Could you check a few things on this model? Use its own coordinates, in mm. A direction names the side the tool comes from. Give positions to 0.01 mm unless a question says otherwise; leave off trailing zeros. Write each loop counter-clockwise with the first axis right and the second up, starting at its lowest first coordinate (ties: lowest second). Pieces come first, ordered by that corner, then holes. Notation, with made-up numbers: (16.25, 8) - (34.25, 8) arc R23 ccw to (34.25, 27) - close; hole circle Ø2 at (42, 50.5). An arc over 180 degrees is marked (long way). Answer in a Markdown table with one row per item.
from build123d import *

# Parameters (mm, degrees)
BOSS_EXTRUDE1_DEPTH          = 6
CHAMFER1_SIZE                = 5
BOSS_EXTRUDE2_DEPTH          = 3
CHAMFER2_SIZE                = 3
SKETCH3_R                    = 2.55
CUT_EXTRUDE1_DEPTH           = 72.316197319
BOSS_EXTRUDE3_START          = 6
SKETCH4_R                    = 5
SKETCH4_R_2                  = 2.55
BOSS_EXTRUDE3_DEPTH          = 6
CHAMFER3_SIZE                = 1
CHAMFER4_SIZE                = 0.5
SKETCH5_R                    = 4.1
CUT_EXTRUDE2_DEPTH           = 5
SKETCH6_R                    = 2.6
CUT_EXTRUDE3_DEPTH           = 10
SKETCH7_R                    = 5
CUT_EXTRUDE4_DEPTH           = 2.8
CUT_EXTRUDE4_DRAFT           = -45
CUT_EXTRUDE4_PROFILE_2_DEPTH = 2.8
CUT_EXTRUDE4_PROFILE_2_DRAFT = -45
CUT_EXTRUDE4_PROFILE_3_DEPTH = 2.8
CUT_EXTRUDE4_PROFILE_3_DRAFT = -45
CUT_EXTRUDE4_PROFILE_4_DEPTH = 2.8
CUT_EXTRUDE4_PROFILE_4_DRAFT = -45
FILLET1_R                    = 2
CUT_EXTRUDE5_START           = -3
SKETCH8_W                    = 20
SKETCH8_H                    = 10
CUT_EXTRUDE5_DEPTH           = 10
CHAMFER5_SIZE                = 2
SKETCH9_R                    = 1.55
SKETCH9_W                    = 3
SKETCH9_H                    = 10
CUT_EXTRUDE6_DEPTH           = 10


with BuildPart() as part:
    # Sketch1 → Boss-Extrude1 (new body)
    with BuildSketch(Plane(origin=(0, 0, 0), x_dir=(1, 0, 0), z_dir=(0, 1, 0))):
        with BuildLine():
            Line((-32, -55), (32, -55))
            ThreePointArc((32, -55), (41.192388155, -51.192388155), (45, -42))
            Line((45, -42), (45, 42))
            ThreePointArc((45, 42), (41.192388155, 51.192388155), (32, 55))
            Line((32, 55), (-32, 55))
            ThreePointArc((-32, 55), (-41.192388155, 51.192388155), (-45, 42))
            Line((-45, 42), (-45, -42))
            ThreePointArc((-45, -42), (-41.192388155, -51.192388155), (-32, -55))
        make_face()
    extrude(amount=BOSS_EXTRUDE1_DEPTH)

    # Chamfer1
    chamfer1_edges = [part.edges().sort_by_distance(p)[0] for p in [
        (45, 0, 0),
        (41.192388155, 0, 51.192388155),
        (0, 0, 55),
        (-41.192388155, 0, 51.192388155),
        (-45, 0, 0),
        (-41.192388155, 0, -51.192388155),
        (0, 0, -55),
        (41.192388155, 0, -51.192388155),
    ]]
    chamfer(chamfer1_edges, length=CHAMFER1_SIZE)

    # Sketch2 → Boss-Extrude2 (add)
    with BuildSketch(Plane(origin=(0, 6, 0), x_dir=(1, 0, 0), z_dir=(0, 1, 0))):
        with BuildLine():
            ThreePointArc((-37.9, -42), (-36.171930009, -46.171930009), (-32, -47.9))
            Line((-32, -47.9), (32, -47.9))
            ThreePointArc((32, -47.9), (36.171930009, -46.171930009), (37.9, -42))
            Line((37.9, -42), (37.9, -21))
            Line((37.9, -21), (41.9, -21))
            Line((41.9, -21), (41.9, -42))
            ThreePointArc((41.9, -42), (39.000357134, -49.000357134), (32, -51.9))
            Line((32, -51.9), (-32, -51.9))
            ThreePointArc((-32, -51.9), (-39.000357134, -49.000357134), (-41.9, -42))
            Line((-41.9, -42), (-41.9, -21))
            Line((-41.9, -21), (-37.9, -21))
            Line((-37.9, -21), (-37.9, -42))
        make_face()
        with BuildLine():
            ThreePointArc((-41.9, 42), (-39.000357134, 49.000357134), (-32, 51.9))
            Line((-32, 51.9), (32, 51.9))
            ThreePointArc((32, 51.9), (39.000357134, 49.000357134), (41.9, 42))
            Line((41.9, 42), (41.9, 21))
            Line((41.9, 21), (37.9, 21))
            Line((37.9, 21), (37.9, 42))
            ThreePointArc((37.9, 42), (36.171930009, 46.171930009), (32, 47.9))
            Line((32, 47.9), (-32, 47.9))
            ThreePointArc((-32, 47.9), (-36.171930009, 46.171930009), (-37.9, 42))
            Line((-37.9, 42), (-37.9, 21))
            Line((-37.9, 21), (-41.9, 21))
            Line((-41.9, 21), (-41.9, 42))
        make_face()
    extrude(amount=BOSS_EXTRUDE2_DEPTH)

    # Chamfer2
    chamfer2_edges = [part.edges().sort_by_distance(p)[0] for p in [
        (37.9, 9, 31.5),
        (36.171930009, 9, 46.171930009),
        (0, 9, 47.9),
        (-36.171930009, 9, 46.171930009),
        (-37.9, 9, 31.5),
        (-37.9, 9, -31.5),
        (-36.171930009, 9, -46.171930009),
        (0, 9, -47.9),
        (36.171930009, 9, -46.171930009),
        (37.9, 9, -31.5),
    ]]
    chamfer(chamfer2_edges, length=CHAMFER2_SIZE - 0.0001)  # a hair under: the kernel refuses the full size

    # Sketch3 → Cut-Extrude1 (cut, through all)
    with BuildSketch(Plane(origin=(0, 6, 0), x_dir=(1, 0, 0), z_dir=(0, 1, 0))):
        with Locations(Location((-25, 30.5, 0), (0, 0, 270))):
            Circle(SKETCH3_R)
        with Locations(Location((25, 30.5, 0), (0, 0, 90))):
            Circle(SKETCH3_R)
        with Locations(Location((25, -30.5, 0), (0, 0, 270))):
            Circle(SKETCH3_R)
        with Locations(Location((-25, -30.5, 0), (0, 0, 90))):
            Circle(SKETCH3_R)
    extrude(amount=-CUT_EXTRUDE1_DEPTH, mode=Mode.SUBTRACT)

    # Sketch4 → Boss-Extrude3 (add)
    # profile 1 of 4: a face of its own
    with BuildSketch(Plane(origin=(0, 6, 0), x_dir=(1, 0, 0), z_dir=(0, 1, 0)).offset(BOSS_EXTRUDE3_START)):
        with Locations(Location((-25, -30.5, 0), (0, 0, 90))):
            Circle(SKETCH4_R)
        with Locations(Location((-25, -30.5, 0), (0, 0, 270))):
            Circle(SKETCH4_R_2, mode=Mode.SUBTRACT)
    # profile 2 of 4: a face of its own
    with BuildSketch(Plane(origin=(0, 6, 0), x_dir=(1, 0, 0), z_dir=(0, 1, 0)).offset(BOSS_EXTRUDE3_START)):
        with Locations(Location((25, -30.5, 0), (0, 0, 90))):
            Circle(SKETCH4_R)
        with Locations(Location((25, -30.5, 0), (0, 0, 270))):
            Circle(SKETCH4_R_2, mode=Mode.SUBTRACT)
    # profile 3 of 4: a face of its own
    with BuildSketch(Plane(origin=(0, 6, 0), x_dir=(1, 0, 0), z_dir=(0, 1, 0)).offset(BOSS_EXTRUDE3_START)):
        with Locations(Location((-25, 30.5, 0), (0, 0, 90))):
            Circle(SKETCH4_R)
        with Locations(Location((-25, 30.5, 0), (0, 0, 270))):
            Circle(SKETCH4_R_2, mode=Mode.SUBTRACT)
    # profile 4 of 4: a face of its own
    with BuildSketch(Plane(origin=(0, 6, 0), x_dir=(1, 0, 0), z_dir=(0, 1, 0)).offset(BOSS_EXTRUDE3_START)):
        with Locations(Location((25, 30.5, 0), (0, 0, 90))):
            Circle(SKETCH4_R)
        with Locations(Location((25, 30.5, 0), (0, 0, 270))):
            Circle(SKETCH4_R_2, mode=Mode.SUBTRACT)
    extrude(amount=-BOSS_EXTRUDE3_DEPTH)

    # Chamfer3
    chamfer3_edges = [part.edges().sort_by_distance(p)[0] for p in [
        (-25, 6, 35.5),
        (25, 6, 35.5),
        (-25, 6, -25.5),
        (25, 6, -25.5),
    ]]
    chamfer(chamfer3_edges, length=CHAMFER3_SIZE)

    # Chamfer4
    chamfer4_edges = [part.edges().sort_by_distance(p)[0] for p in [
        (-25, 12, 35.5),
        (25, 12, 35.5),
        (-25, 12, -25.5),
        (25, 12, -25.5),
    ]]
    chamfer(chamfer4_edges, length=CHAMFER4_SIZE)

    # Sketch5 → Cut-Extrude2 (cut)
    with BuildSketch(Plane.XZ):
        with Locations(Location((-25, 30.5, 0), (0, 0, 270))):
            Circle(SKETCH5_R)
        with Locations(Location((25, 30.5, 0), (0, 0, 270))):
            Circle(SKETCH5_R)
        with Locations(Location((-25, -30.5, 0), (0, 0, 270))):
            Circle(SKETCH5_R)
        with Locations(Location((25, -30.5, 0), (0, 0, 270))):
            Circle(SKETCH5_R)
    extrude(amount=-CUT_EXTRUDE2_DEPTH, mode=Mode.SUBTRACT)

    # Sketch6 → Cut-Extrude3 (cut)
    with BuildSketch(Plane(origin=(0, 6, 0), x_dir=(1, 0, 0), z_dir=(0, 1, 0))):
        with Locations(Location((-32, 42, 0), (0, 0, 270))):
            Circle(SKETCH6_R)
        with Locations(Location((32, 42, 0), (0, 0, 270))):
            Circle(SKETCH6_R)
        with Locations(Location((32, -42, 0), (0, 0, 270))):
            Circle(SKETCH6_R)
        with Locations(Location((-32, -42, 0), (0, 0, 270))):
            Circle(SKETCH6_R)
    extrude(amount=-CUT_EXTRUDE3_DEPTH, mode=Mode.SUBTRACT)


with BuildPart() as cut_extrude4_tool:
    # Sketch7 → Cut-Extrude4 (with draft: the straight prism first)
    with BuildSketch(Plane.XZ):
        with Locations((32, 42)):
            Circle(SKETCH7_R)
    extrude(amount=-CUT_EXTRUDE4_DEPTH)
    # Cut-Extrude4: the draft: its side faces are tilted about the plane it starts from
    cut_extrude4_sides = [cut_extrude4_tool.faces().sort_by_distance(p)[0] for p in [
        (27, 1.4, 42),
    ]]
    draft(cut_extrude4_sides, Plane.XZ, CUT_EXTRUDE4_DRAFT)


with BuildPart() as part_1:
    add(part.part)

    # Cut-Extrude4: cut by cut_extrude4_tool
    add(cut_extrude4_tool.part, mode=Mode.SUBTRACT)


with BuildPart() as cut_extrude4_profile_2_tool:
    # Sketch7 → Cut-Extrude4 profile 2 (with draft: the straight prism first)
    with BuildSketch(Plane.XZ):
        with Locations((-32, 42)):
            Circle(SKETCH7_R)
    extrude(amount=-CUT_EXTRUDE4_PROFILE_2_DEPTH)
    # Cut-Extrude4 profile 2: the draft: its side faces are tilted about the plane it starts from
    cut_extrude4_profile_2_sides = [cut_extrude4_profile_2_tool.faces().sort_by_distance(p)[0] for p in [
        (-37, 1.4, 42),
    ]]
    draft(cut_extrude4_profile_2_sides, Plane.XZ, CUT_EXTRUDE4_PROFILE_2_DRAFT)


with BuildPart() as part_2:
    add(part_1.part)

    # Cut-Extrude4 profile 2: cut by cut_extrude4_profile_2_tool
    add(cut_extrude4_profile_2_tool.part, mode=Mode.SUBTRACT)


with BuildPart() as cut_extrude4_profile_3_tool:
    # Sketch7 → Cut-Extrude4 profile 3 (with draft: the straight prism first)
    with BuildSketch(Plane.XZ):
        with Locations((-32, -42)):
            Circle(SKETCH7_R)
    extrude(amount=-CUT_EXTRUDE4_PROFILE_3_DEPTH)
    # Cut-Extrude4 profile 3: the draft: its side faces are tilted about the plane it starts from
    cut_extrude4_profile_3_sides = [cut_extrude4_profile_3_tool.faces().sort_by_distance(p)[0] for p in [
        (-37, 1.4, -42),
    ]]
    draft(cut_extrude4_profile_3_sides, Plane.XZ, CUT_EXTRUDE4_PROFILE_3_DRAFT)


with BuildPart() as part_3:
    add(part_2.part)

    # Cut-Extrude4 profile 3: cut by cut_extrude4_profile_3_tool
    add(cut_extrude4_profile_3_tool.part, mode=Mode.SUBTRACT)


with BuildPart() as cut_extrude4_profile_4_tool:
    # Sketch7 → Cut-Extrude4 profile 4 (with draft: the straight prism first)
    with BuildSketch(Plane.XZ):
        with Locations((32, -42)):
            Circle(SKETCH7_R)
    extrude(amount=-CUT_EXTRUDE4_PROFILE_4_DEPTH)
    # Cut-Extrude4 profile 4: the draft: its side faces are tilted about the plane it starts from
    cut_extrude4_profile_4_sides = [cut_extrude4_profile_4_tool.faces().sort_by_distance(p)[0] for p in [
        (27, 1.4, -42),
    ]]
    draft(cut_extrude4_profile_4_sides, Plane.XZ, CUT_EXTRUDE4_PROFILE_4_DRAFT)


with BuildPart() as part_4:
    add(part_3.part)

    # Cut-Extrude4 profile 4: cut by cut_extrude4_profile_4_tool
    add(cut_extrude4_profile_4_tool.part, mode=Mode.SUBTRACT)

    # Fillet1
    fillet1_edges = [part_4.edges().sort_by_distance(p)[0] for p in [
        (39.9, 6, 21),
        (-39.9, 6, 21),
        (-39.9, 6, -21),
        (39.9, 6, -21),
    ]]
    fillet(fillet1_edges, radius=FILLET1_R)

    # Sketch8 → Cut-Extrude5 (cut)
    with BuildSketch(Plane.XZ.offset(CUT_EXTRUDE5_START)):
        with Locations((0, -10.11628608)):
            Rectangle(SKETCH8_W, SKETCH8_H)
    extrude(amount=-CUT_EXTRUDE5_DEPTH, mode=Mode.SUBTRACT)

    # Chamfer5
    chamfer5_edges = [part_4.edges().sort_by_distance(p)[0] for p in [
        (-10, 6, -10.11628608),
        (10, 6, -10.11628608),
    ]]
    chamfer(chamfer5_edges, length=CHAMFER5_SIZE)

    # Sketch9 → Cut-Extrude6 (cut)
    with BuildSketch(Plane(origin=(0, 3, 0), x_dir=(1, 0, 0), z_dir=(0, 1, 0))):
        with Locations(Location((0, 10.11628608, 0), (0, 0, 270))):
            Circle(SKETCH9_R)
        with Locations((-8.5, 10.11628608)):
            Rectangle(SKETCH9_W, SKETCH9_H)
        with Locations((8.5, 10.11628608)):
            Rectangle(SKETCH9_W, SKETCH9_H)
    extrude(amount=-CUT_EXTRUDE6_DEPTH, mode=Mode.SUBTRACT)


solid = part_4.part
1) Imagine slicing it at B-B (z = -17.5). List the corners of the cut face in (x, y) for me, then the cut area to 3 significant figures.
Check values:
| item | result |
|---|---|
| outline | (-45, 5) - (-40, 0) - (40, 0) - (45, 5) - (45, 6) - (-45, 6) - close |
| area | 515 mm2 |
2) Imagine slicing it at D-D (x = 25). State how many separate pieces and enclosed holes the cut face has, then the cut area to 3 significant figures.
Check values:
| item | result |
|---|---|
| separate pieces | 3 |
| enclosed holes | 0 |
| area | 618 mm2 |
3) Will these pins go through, and if not, where does the flat tip stop? P1, Ø1.5, axis at y = 2, z = -10, coming from the -X side; P2, Ø0.9, axis at y = 7.5, z = 33.5, coming from the -X side; P3, Ø3, axis at x = 34, y = 7, coming from the +Z side; P4, Ø4, axis at x = 32, z = -42, coming from the +Y side.
Check values:
| item | result |
|---|---|
| P1 | stops at x = -42.75 |
| P2 | stops at x = -41.9 |
| P3 | stops at z = 54.97 |
| P4 | passes through |
4) We'd pull the mould along X, two halves only. Please class faces 1 (the face through (-23.06, 12, 28.56)), 2 (the face through (-42, 2, -1)), 3 (the face through (25.1, 5, -33.2)): +X half, -X half, draft (parallel to the pull), parting line (faces both ways), or undercut.
Check values:
| item | result |
|---|---|
| face 1 | draft |
| face 2 | -X half |
| face 3 | undercut |
5) If I drill on line 1 (Z direction, x = 31.5, y = 2.5); line 2 (X direction, y = 4.85, z = 42); line 3 (X direction, y = 3.6, z = -30.5), over which ranges is the centre line in solid material (lowest first)?
Check values:
| item | result |
|---|---|
| line 1 | z = -52.5 to -44.55, -39.45 to 39.45, 44.55 to 52.5 |
| line 2 | x = -44.85 to -34.6, -29.4 to 29.4, 34.6 to 44.85 |
| line 3 | x = -43.6 to -29.1, -20.9 to 20.9, 29.1 to 43.6 |
6) On a 3-axis mill with a long thin cutter (end or side, diameter ignored), from which of +Z, -Z, +X, -X, +Y, -Y can I reach the whole of each face in a straight line? I mean faces 4 (the face through (7, 2, -10)), 5 (the face through (-41.9, 7, 31)), 6 (the face through (39.4, 7.5, -30.3)). Say none if no direction works.
Check values:
| item | result |
|---|---|
| face 4 | +Y, -Y |
| face 5 | +Z, -Z, -X, +Y |
| face 6 | +Y |
